Build history of the part. All positions in model axes, mm. A direction names the side the tool comes from. Give positions to 0.01 mm unless a question says otherwise; leave off trailing zeros. Order: outer loops, then holes, each group sorted by start corner. A loop starts at its lowest first (then second) coordinate and runs counter-clockwise, first axis right, second up. Notation, with made-up numbers: (25, 84.5) -> (73, 84.5) arc R21 cw to (73, 119.5) -> close; hole circle Ø4 at (70.25, 14.25). An arc over 180 degrees is marked (long way). One line per item, written item: value. Start each with the question number.
(1) Pin check, flat tips, straight feed: pin 1 (7.5 mm diameter, centred on y = -18, z = 81, fed in from -X); pin 2 (12.5 mm diameter, centred on y = -15, z = 5.5, fed in from -X); pin 3 (20.5 mm diameter, centred on x = -16, y = -38, fed in from -Z). Stop position of each tip, or through.
(2) Saw through at A-A on x = -22. Give the cut face in (y, z).
(3) Which spindle directions (+Z, -Z, +X, -X, +Y, -Y) get a long thin tool onto all of the face, cutting with end or side? Do faces 5 (the flat face through (0, -38, -47.56)), 6 (the flat face through (0, -38, 42.59)), 7 (the flat face through (61.599, -13, -2)), 8 (the flat face through (-62.354, -13, -2)). Say none if no direction does.
(4) Probe line 1 (Z direction, x = -44.5, y = -18); line 2 (Z direction, x = 48.5, y = -13); line 3 (X direction, y = -3.5, z = 82.5). List the from-to ranges inside material, lowest first.
(5) Saw through at C-C on y = -13. Give the cut face in (x, z), plus the area to 3 significant figures.
(6) Saw through at D-D on x = 2. Give the cut face in (y, z).
(7) Two-plate mould, pull along Z, no slides. Class faces 1 (the flat face through (-1, -13, -58.591)), 2 (the flat face through (37, -13, 101.428)), 3 (the flat face through (-39, -12, 103.429)), 4 (the flat face through (62.547, -13, 114)): +Z half, -Z half, draft (parallel to the pull), parting line (faces both ways), or undercut.
(8) Saw through at B-B on z = 38.5. Give the cut face in (x, y).
```python
from build123d import *

# Parameters (mm, degrees)
F0_W     = 123.9526234567
F0_H     = 115.1683554053
F1_DEPTH = 25.4
F2_W     = 100.4445962608
F2_H     = 90.1500321925
F3_DEPTH = 50.8
F4_W     = 26.1205909774
F4_H     = 25.0108242035
F5_DEPTH = 127
F6_W     = 25.0108242035
F6_H     = 23.5706527233
F7_DEPTH = 50.8
F8_W     = 25.0108242035
F8_H     = 25.5720127821
F9_DEPTH = 50.8


with BuildPart() as f1:
    # F0 (on Front) → F1 (new body)
    with BuildSketch(Plane.XZ):
        with Locations((-0.3773439676, -1.0064095259)):
            Rectangle(F0_W, F0_H)
    extrude(amount=F1_DEPTH)

    # F2 (on Front) → F3 (join)
    with BuildSketch(Plane.XZ):
        with Locations((0.9114388376, -2.4853553623)):
            Rectangle(F2_W, F2_H)
    extrude(amount=F3_DEPTH)

    # F4 (on Top) → F5 (join)
    with BuildSketch(Plane.XY):
        with Locations((-1.3128877617, -12.5054121017)):
            Rectangle(F4_W, F4_H)
    extrude(amount=F5_DEPTH)

    # F6 (on face) → F7 (join)
    with BuildSketch(Plane(origin=(-14.3731832504, 0, 0), x_dir=(0, -1, 0), z_dir=(-1, 0, 0))):
        with Locations((12.5054121017, 115.2146736383)):
            Rectangle(F6_W, F6_H)
    extrude(amount=F7_DEPTH)

    # F8 (on face) → F9 (join)
    with BuildSketch(Plane.YZ.offset(11.7474077269)):
        with Locations((-12.5054121017, 114.213993609)):
            Rectangle(F8_W, F8_H)
    extrude(amount=F9_DEPTH)


solid = f1.part
```
Results below:
1. pin 1: stops at x = -14.37
1. pin 2: stops at x = -62.35
1. pin 3: stops at z = -47.56
2. outline: (-50.8, -47.56) -> (-25.4, -47.56) -> (-25.4, -58.59) -> (0, -58.59) -> (0, 56.58) -> (-25.4, 56.58) -> (-25.4, 42.59) -> (-50.8, 42.59) -> close; (-25.01, 103.43) -> (0, 103.43) -> (0, 127) -> (-25.01, 127) -> close
3. face 5: -Z, +X, -X, -Y
3. face 6: +Z, +X, -X, -Y
3. face 7: -Z, +X, +Y, -Y
3. face 8: -Z, -X, +Y, -Y
4. line 1: z = -58.59 to 56.58, 103.43 to 127
4. line 2: z = -58.59 to 56.58, 101.43 to 127
4. line 3: x = -14.37 to 11.75
5. outline: (-65.17, 103.43) -> (-14.37, 103.43) -> (-14.37, 56.58) -> (-62.35, 56.58) -> (-62.35, -58.59) -> (61.6, -58.59) -> (61.6, 56.58) -> (11.75, 56.58) -> (11.75, 101.43) -> (62.55, 101.43) -> (62.55, 127) -> (-65.17, 127) -> close
5. area: 18,600 mm²
6. outline: (-50.8, -47.56) -> (-25.4, -47.56) -> (-25.4, -58.59) -> (0, -58.59) -> (0, 127) -> (-25.01, 127) -> (-25.01, 56.58) -> (-25.4, 56.58) -> (-25.4, 42.59) -> (-50.8, 42.59) -> close
7. face 1: -Z half
7. face 2: undercut
7. face 3: undercut
7. face 4: draft
8. outline: (-62.35, -25.4) -> (-49.31, -25.4) -> (-49.31, -50.8) -> (51.13, -50.8) -> (51.13, -25.4) -> (61.6, -25.4) -> (61.6, 0) -> (-62.35, 0) -> close
